Design review of the part shown in the three views and the two pictorial views. Dimensions are in mm from the part's minimum x, y and z. Round coordinates to 2 decimals unless told otherwise and drop trailing zeros. Loops run counter-clockwise (first coordinate to the right, second up) from the corner with the lowest first, then second, coordinate; pieces in that order, holes last.
1) Insertion check: pin 1 (4 mm diameter, centred on x = 19, z = 7.5, fed in from -Y). The pin has a flat end and moves straight along its axis. Give the tip position at first contact, or say it passes through.
2) Wall thickness on L1, parallel to Z at x = 30, y = 2 (1 decimal); L2, parallel to X at y = 2.05, z = 12; L3, parallel to Z at x = 23, y = 1.2: over which ranges is each line inside the solid? List them lowest first.
3) Take a section at A-A (z = 25.4). State the section outline as (x, y) points (3 decimals), then the cut area to 3 significant figures.
4) Take a section at B-B (x = 7). State the section outline as (y, z) points (1 decimal).
5) Take a section at D-D (x = 27). State the section outline as (y, z) points (1 decimal).
6) Take a section at C-C (y = 2.05). Give the number of separate pieces and of enclosed holes in the cut face, then the cut area to 3 significant figures.
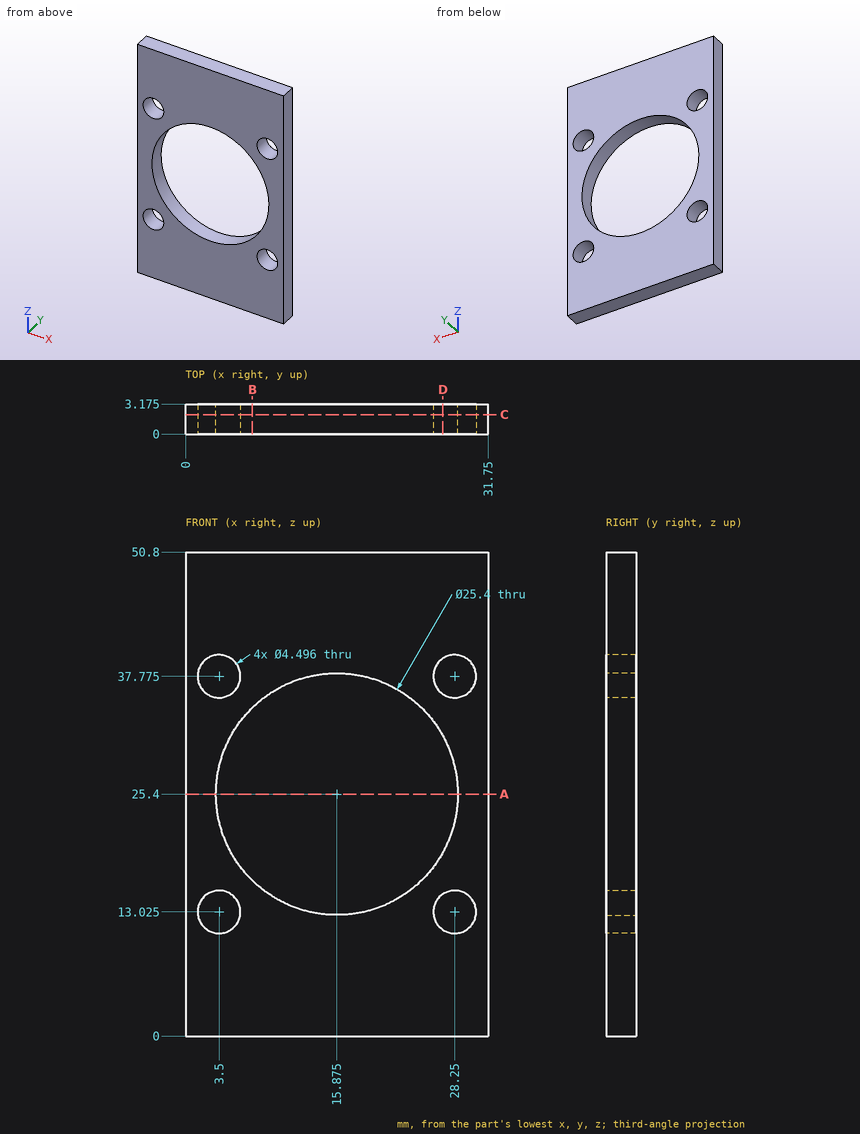
Response:
1. pin 1: stops at y = 0
2. L1: z = 0 to 11.6, 14.4 to 36.4, 39.2 to 50.8
2. L2: x = 0 to 1.5, 5.5 to 26.25, 30.25 to 31.75
2. L3: z = 0 to 14.89, 35.91 to 50.8
3. outline: (0, 0) - (3.175, 0) - (3.175, 3.175) - (0, 3.175) - close; (28.575, 0) - (31.75, 0) - (31.75, 3.175) - (28.575, 3.175) - close
3. area: 20.2 mm2
4. outline: (0, 0) - (3.2, 0) - (3.2, 16.3) - (0, 16.3) - close; (0, 34.5) - (3.2, 34.5) - (3.2, 50.8) - (0, 50.8) - close
5. outline: (0, 0) - (3.2, 0) - (3.2, 11.2) - (0, 11.2) - close; (0, 14.9) - (3.2, 14.9) - (3.2, 19.3) - (0, 19.3) - close; (0, 31.5) - (3.2, 31.5) - (3.2, 35.9) - (0, 35.9) - close; (0, 39.6) - (3.2, 39.6) - (3.2, 50.8) - (0, 50.8) - close
6. separate pieces: 1
6. enclosed holes: 5
6. area: 1,040 mm2
